Verification items for the finished model (mm, model axes). Face numbers are marked on the shaded views. Give positions to 0.01 mm unless a question says otherwise; leave off trailing zeros. Order: outer loops, then holes, each group sorted by start corner. A loop starts at its lowest first (then second) coordinate and runs counter-clockwise, first axis right, second up. Notation, with made-up numbers: (9.5, -19.5) - (44.5, -19.5) arc R26 cw to (44.5, 7.5) - close; hole circle Ø5 at (5, -30.75). An arc over 180 degrees is marked (long way). Answer as a JSON object with one key per item and string values.
```python
from build123d import *

# Parameters (mm, degrees)
F0_R     = 52.5018
F0_R_2   = 30.1625
F1_DEPTH = 152.4
F3_DEPTH = 52.5028


# Not quite as in the source:
# - a feature names something its author has since deleted; it is built from what else it names


with BuildPart() as f1:
    # F0 (on Top) → F1 (new body)
    with BuildSketch(Plane.XY):
        Circle(F0_R)
        Circle(F0_R_2, mode=Mode.SUBTRACT)
    extrude(amount=-F1_DEPTH)

    # F2 (on Right) → F3 (cut, through all)
    with BuildSketch(Plane.YZ):
        with BuildLine():
            ThreePointArc((0.25, -49.3), (0.1767766953, -49.1232233047), (0, -49.05))
            Line((0, -49.05), (0, -49.55))
            ThreePointArc((0, -49.55), (0.1767766953, -49.4767766953), (0.25, -49.3))
        make_face()
        with BuildLine():
            ThreePointArc((0.25, -103.1), (0.1767766953, -102.9232233047), (0, -102.85))
            Line((0, -102.85), (0, -103.35))
            ThreePointArc((0, -103.35), (0.1767766953, -103.2767766953), (0.25, -103.1))
        make_face()
        with BuildLine():
            Line((0, -103.35), (0, -102.85))
            ThreePointArc((0, -102.85), (-0.25, -103.1), (0, -103.35))
        make_face()
        with BuildLine():
            ThreePointArc((0.25, -100.1), (0.1767766953, -99.9232233047), (0, -99.85))
            Line((0, -99.85), (0, -100.35))
            ThreePointArc((0, -100.35), (0.1767766953, -100.2767766953), (0.25, -100.1))
        make_face()
        with BuildLine():
            Line((0, -100.35), (0, -99.85))
            ThreePointArc((0, -99.85), (-0.25, -100.1), (0, -100.35))
        make_face()
        with BuildLine():
            ThreePointArc((0.25, -52.3), (0.1767766953, -52.1232233047), (0, -52.05))
            Line((0, -52.05), (0, -52.55))
            ThreePointArc((0, -52.55), (0.1767766953, -52.4767766953), (0.25, -52.3))
        make_face()
        with BuildLine():
            Line((0, -52.55), (0, -52.05))
            ThreePointArc((0, -52.05), (-0.25, -52.3), (0, -52.55))
        make_face()
        with BuildLine():
            Line((0, -49.55), (0, -49.05))
            ThreePointArc((0, -49.05), (-0.25, -49.3), (0, -49.55))
        make_face()
    extrude(amount=-F3_DEPTH, mode=Mode.SUBTRACT)


solid = f1.part
```
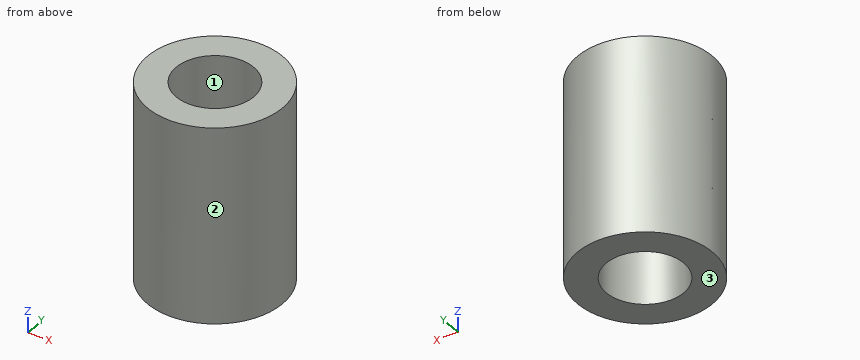
(1) Section check B-B (y = 9). Record the cut outline in (x, z).
Computed values:
{"outline": "(-51.72, -152.4) - (-28.79, -152.4) - (-28.79, 0) - (-51.72, 0) - close; (28.79, -152.4) - (51.72, -152.4) - (51.72, 0) - (28.79, 0) - close"}
(2) Release check for a two-part mould opening along Y. For the marked faces 1, 2 and 3 record: pulls with the +Y half, pulls with the -Y half, needs draft (parallel to the pull), parting line crosses it, or undercut.
Computed values:
{"face 1": "undercut", "face 2": "parting line crosses it", "face 3": "needs draft"}
(3) Section check C-C (z = -127). Record the cut outline in (x, y) (1 decimal).
Computed values:
{"outline": "circle Ø105 at (0, 0); hole circle Ø60.3 at (0, 0)"}
(4) Section check D-D (y = 39). Record the cut outline in (x, z).
Computed values:
{"outline": "(-35.15, -152.4) - (35.15, -152.4) - (35.15, 0) - (-35.15, 0) - close"}
(5) Material ranges on line 1 along Y through (x, z) = (0, -39.5); line 2 along X through (y, z) = (-12.5, -113), recorded low to high. Write a range as [from, to].
Computed values:
{"line 1": "y = [-52.5, -30.16], [30.16, 52.5]", "line 2": "x = [-50.99, -27.45], [27.45, 50.99]"}
(6) Gauge pin test, flat ends, axial feed: pin 1 Ø1 at (y, z) = (-20, -91.5) entering from +X; pin 2 Ø10 at (x, z) = (34.5, -75) entering from +Y; pin 3 Ø3 at (x, z) = (-36, -16) entering from -Y. Record the tip position at first contact, or that the pin passes through.
Computed values:
{"pin 1": "stops at x = 48.75", "pin 2": "stops at y = 43.43", "pin 3": "stops at y = -39.58"}
(7) Section check A-A (x = 0). Record the cut outline in (y, z), then the cut area to 3 significant figures.
Computed values:
{"outline": "(-52.5, -152.4) - (-30.16, -152.4) - (-30.16, 0) - (-52.5, 0) - close; (30.16, -152.4) - (52.5, -152.4) - (52.5, 0) - (30.16, 0) - close", "area": "6,810 mm²"}
